Here's how the part is built. I have some questions about the finished solid (model axes, mm). A direction names the side the tool comes from. Coordinates: 2 decimals unless noted, no trailing zeros. Write each loop counter-clockwise with the first axis right and the second up, starting at its lowest first coordinate (ties: lowest second). Pieces come first, ordered by that corner, then holes. Notation, with made-up numbers: (-13, -33) -> (15, -33) arc R10 cw to (15, -15) -> close; hole circle Ø9 at (77.5, 8). An arc over 180 degrees is marked (long way). Use a Markdown table: item, result. Add a question column.
Item 1: Imagine slicing it at A-A, the plane y = -16.5. Write out the boundary of the cut face in (x, z) (3 decimals).
Item 2: On a 3-axis mill with a long thin cutter (end or side, diameter ignored), from which of +Z, -Z, +X, -X, +Y, -Y can I reach the whole of each face in a straight line? I mean faces 1 (the flat face through (2, -22.225, -33)), 2 (the flat face through (16, 0, -47.625)). Say none if no direction works.
Item 3: Imagine slicing it at C-C, the plane x = 20. Write out the boundary of the cut face in (y, z) (3 decimals), and give its area (3 significant figures).
Item 4: Imagine slicing it at B-B, the plane z = -35.5. Write out the boundary of the cut face in (x, y) (3 decimals), and give its area (3 significant figures).
Item 5: Will this pin go through, and if not, where does the flat tip stop? pin 1 Ø6 at (x, z) = (8.5, -13.5) entering from -Y.
Item 6: If I drill on line 1 along X through (y, z) = (17, -3) (3 decimals); line 2 along Z through (x, y) = (24.75, -1) (3 decimals); line 3 along Z through (x, y) = (2.5, -3.5), over which ranges is the centre line in solid material (lowest first)? Write a range as from..to.
```python
from build123d import *

# Parameters (mm, degrees)
SKETCH3_W = 3.175
SKETCH3_H = 44.45
FILLET1_R = 3.175
FILLET2_R = 6.35


with BuildPart() as part:
    # Sweep1: sweep along a path in Sketch4
    with BuildLine(Plane(origin=(0, 0, 0), x_dir=(1, 0, 0), z_dir=(0, 1, 0))) as sweep1_path:
        Line((0, 0), (0, 50.8))
        Line((0, 50.8), (25.4, 50.8))
    # Sketch3 → Sweep1 (sweep)
    with BuildSketch(Plane.XY):
        with Locations((1.5875, 0)):
            Rectangle(SKETCH3_W, SKETCH3_H)
    sweep(path=sweep1_path.line, transition=Transition.RIGHT)

    # Fillet1
    fillet1_edges = [part.edges().sort_by_distance(p)[0] for p in [
        (3.175, 0, -47.625),
    ]]
    fillet(fillet1_edges, radius=FILLET1_R)

    # Fillet2
    fillet2_edges = [part.edges().sort_by_distance(p)[0] for p in [
        (0, 0, -50.8),
    ]]
    fillet(fillet2_edges, radius=FILLET2_R)


solid = part.part
```
Ans:
| question | item | result |
|---|---|---|
| 1 | outline | (0, -44.45) arc R6.35 ccw to (6.35, -50.8) -> (25.4, -50.8) -> (25.4, -47.625) -> (6.35, -47.625) arc R3.175 cw to (3.175, -44.45) -> (3.175, 0) -> (0, 0) -> close |
| 2 | face 1 | +Z, -Z, +X, -X, -Y |
| 2 | face 2 | +Z, +X, +Y, -Y |
| 3 | outline | (-22.225, -50.8) -> (22.225, -50.8) -> (22.225, -47.625) -> (-22.225, -47.625) -> close |
| 3 | area | 141 mm^2 |
| 4 | outline | (0, -22.225) -> (3.175, -22.225) -> (3.175, 22.225) -> (0, 22.225) -> close |
| 4 | area | 141 mm^2 |
| 5 | pin 1 | passes through |
| 6 | line 1 | x = 0..3.175 |
| 6 | line 2 | z = -50.8..-47.625 |
| 6 | line 3 | z = -49.5..0 |
